Build history of the part. All positions in model axes, mm. A direction names the side the tool comes from. Round coordinates to 2 decimals unless told otherwise and drop trailing zeros. Order: outer loops, then holes, each group sorted by start corner. A loop starts at its lowest first (then second) coordinate and runs counter-clockwise, first axis right, second up. Notation, with made-up numbers: (-5.75, 50) -> (26.25, 50) arc R13 ccw to (26.25, 66) -> close; hole circle Ø1 at (87, 27.5). An arc over 180 degrees is marked (long way). Answer as a JSON object with one key per item and string values.
from build123d import *

# Parameters (mm, degrees)
BOSS_EXTRUDE1_DEPTH = 4.476
CUT_EXTRUDE1_DEPTH  = 2.413
SKETCH4_R           = 1.65
CUT_EXTRUDE2_DEPTH  = 5.476
SKETCH5_R           = 8.0645
CUT_EXTRUDE3_DEPTH  = 3.175


with BuildPart() as part:
    # Sketch1 → Boss-Extrude1 (new body)
    with BuildSketch(Plane(origin=(0, 0, 0), x_dir=(1, 0, 0), z_dir=(0, 1, 0))):
        Polygon((8.13035809, -26.001312997), (71.63035809, -26.001312997), (71.63035809, -13.301312997), (71.63035809, 15.908687003), (71.63035809, 37.498687003), (8.13035809, 37.498687003), (8.13035809, 22.258687003), (8.13035809, -19.651312997), align=None)
    extrude(amount=BOSS_EXTRUDE1_DEPTH)

    # Sketch2 → Cut-Extrude1 (cut)
    with BuildSketch(Plane(origin=(0, 4.476, 0), x_dir=(1, 0, 0), z_dir=(0, 1, 0))):
        Polygon((64.265579696, 28.926187003), (67.565136484, 28.926187003), (69.214914879, 31.783687003), (67.565136484, 34.641187003), (64.265579696, 34.641187003), (62.615801302, 31.783687003), align=None)
        Polygon((17.144914879, 31.783687003), (15.495136484, 34.641187003), (12.195579696, 34.641187003), (10.545801302, 31.783687003), (12.195579696, 28.926187003), (15.495136484, 28.926187003), align=None)
        Polygon((64.265579696, -23.143812997), (67.565136484, -23.143812997), (69.214914879, -20.286312997), (67.565136484, -17.428812997), (64.265579696, -17.428812997), (62.615801302, -20.286312997), align=None)
        Polygon((12.195579696, -23.143812997), (15.495136484, -23.143812997), (17.144914879, -20.286312997), (15.495136484, -17.428812997), (12.195579696, -17.428812997), (10.545801302, -20.286312997), align=None)
    extrude(amount=-CUT_EXTRUDE1_DEPTH, mode=Mode.SUBTRACT)

    # Sketch4 → Cut-Extrude2 (cut, through all)
    with BuildSketch(Plane(origin=(0, 4.476, 0), x_dir=(1, 0, 0), z_dir=(0, 1, 0))):
        with Locations((65.91535809, 31.783687003)):
            Circle(SKETCH4_R)
        with Locations((13.84535809, 31.783687003)):
            Circle(SKETCH4_R)
        with Locations((65.91535809, -20.286312997)):
            Circle(SKETCH4_R)
        with Locations((13.84535809, -20.286312997)):
            Circle(SKETCH4_R)
    extrude(amount=-CUT_EXTRUDE2_DEPTH, mode=Mode.SUBTRACT)

    # Sketch5 → Cut-Extrude3 (cut)
    with BuildSketch(Plane(origin=(0, 4.476, 0), x_dir=(1, 0, 0), z_dir=(0, 1, 0))):
        with Locations((39.88035809, 5.748687003)):
            Circle(SKETCH5_R)
    extrude(amount=-CUT_EXTRUDE3_DEPTH, mode=Mode.SUBTRACT)


solid = part.part
1) Probe L1, parallel to X at y = 0.8, z = 20.5; L2, parallel to X at y = 3.15, z = -32; L3, parallel to Y at x = 42, z = -8. List the from-to ranges inside material, lowest first. Write a range as from..to.
Checked values:
{"L1": "x = 8.13..12.21, 15.48..64.28, 67.55..71.63", "L2": "x = 8.13..10.67, 17.02..62.74, 69.09..71.63", "L3": "y = 0..1.3"}
2) Cut at A-A, the plane x = 14.5. Give the cut face in (y, z), plus the area to 3 significant figures.
Checked values:
{"outline": "(0, -37.5) -> (4.48, -37.5) -> (4.48, -34.64) -> (2.06, -34.64) -> (2.06, -33.3) -> (0, -33.3) -> close; (0, -30.27) -> (2.06, -30.27) -> (2.06, -28.93) -> (4.48, -28.93) -> (4.48, 17.43) -> (2.06, 17.43) -> (2.06, 18.77) -> (0, 18.77) -> close; (0, 21.8) -> (2.06, 21.8) -> (2.06, 23.14) -> (4.48, 23.14) -> (4.48, 26) -> (0, 26) -> close", "area": "244 mm²"}
3) Which spindle directions (+Z, -Z, +X, -X, +Y, -Y) get a long thin tool onto all of the face, cutting with end or side? Do faces 5 (the face through (63.43, 3.29, 21.7)), 6 (the face through (67.44, 1.05, 20.92)). Say none if no direction does.
Checked values:
{"face 5": "+Y", "face 6": "+Y, -Y"}
4) Cut at B-B, the plane y = 3.2. Count the separate pieces of the cut face and the enclosed holes in it, plus the area to 3 significant figures.
Checked values:
{"separate pieces": "1", "enclosed holes": "5", "area": "3,710 mm²"}
5) Cut at C-C, the plane z = 0.5. Give the cut face in (x, y), plus the area to 3 significant figures.
Checked values:
{"outline": "(8.13, 0) -> (71.63, 0) -> (71.63, 4.48) -> (44.98, 4.48) -> (44.98, 1.3) -> (34.78, 1.3) -> (34.78, 4.48) -> (8.13, 4.48) -> close", "area": "252 mm²"}
6) Pull direction Z, two halves, no side cores. Call faces 1 (the face through (40, 2, -37.499)), 2 (the face through (8.13, 2, -6)), 3 (the face through (39, 2, 26.001)), 4 (the face through (67.3, 2.063, 19)): pulls with the +Z half, pulls with the -Z half, needs draft (parallel to the pull), parting line crosses it, or undercut.
Checked values:
{"face 1": "pulls with the -Z half", "face 2": "needs draft", "face 3": "pulls with the +Z half", "face 4": "undercut"}
7) Cut at D-D, the plane z = -9.5. Give the cut face in (x, y), plus the area to 3 significant figures.
Checked values:
{"outline": "(8.13, 0) -> (71.63, 0) -> (71.63, 4.48) -> (47.02, 4.48) -> (47.02, 1.3) -> (32.74, 1.3) -> (32.74, 4.48) -> (8.13, 4.48) -> close", "area": "239 mm²"}
8) Flat gauge pins, fed straight in: pin 1 Ø1.7 at (x, z) = (67, 20) entering from +Y; pin 2 Ø9.5 at (x, z) = (39.88, -5.75) entering from +Y. Where does each tip first touch, or does it go through?
Checked values:
{"pin 1": "stops at y = 2.06", "pin 2": "stops at y = 1.3"}
